```python
from build123d import *

# Parameters (mm, degrees)
F1_DEPTH      = 6.35
F2_R          = 2.54
F3_DEPTH      = 25.4
F3_DEPTH_BACK = 25.4


with BuildPart() as f1:
    # F0 (on Top) → F1 (new body)
    with BuildSketch(Plane.XY):
        with BuildLine():
            Line((-8.89, -12.7), (8.89, -12.7))
            ThreePointArc((8.89, -12.7), (11.584077, -11.584077), (12.7, -8.89))
            Line((12.7, -8.89), (12.7, 8.89))
            ThreePointArc((12.7, 8.89), (11.584077, 11.584077), (8.89, 12.7))
            Line((8.89, 12.7), (-8.89, 12.7))
            ThreePointArc((-8.89, 12.7), (-11.584077, 11.584077), (-12.7, 8.89))
            Line((-12.7, 8.89), (-12.7, -8.89))
            ThreePointArc((-12.7, -8.89), (-11.584077, -11.584077), (-8.89, -12.7))
        make_face()
    extrude(amount=F1_DEPTH)

    # F2 (on Top) → F3 (cut, two sides)
    with BuildSketch(Plane.XY) as f3_sk:
        with Locations((-6.336518, -6.325952)):
            Circle(F2_R)
        with Locations((6.331818, -6.326862)):
            Circle(F2_R)
        with Locations((6.324662, 6.333847)):
            Circle(F2_R)
        with Locations((-6.33241, 6.329887)):
            Circle(F2_R)
    extrude(amount=F3_DEPTH, mode=Mode.SUBTRACT)
    extrude(f3_sk.sketch, amount=-F3_DEPTH_BACK, mode=Mode.SUBTRACT)


solid = f1.part
```
Here's how the part is built. I have some questions about the finished solid (model axes, mm). Give positions to 0.01 mm unless a question says otherwise; leave off trailing zeros. Write each loop counter-clockwise with the first axis right and the second up, starting at its lowest first coordinate (ties: lowest second). Pieces come first, ordered by that corner, then holes.
(1) Imagine slicing it at B-B, the plane y = 8.5. Write out the boundary of the cut face in (x, z).
Output values:
outline: (-12.7, 0) - (-7.65, 0) - (-7.65, 6.35) - (-12.7, 6.35) - close; (-5.01, 0) - (5, 0) - (5, 6.35) - (-5.01, 6.35) - close; (7.65, 0) - (12.7, 0) - (12.7, 6.35) - (7.65, 6.35) - close
(2) Imagine slicing it at C-C, the plane z = 2.5. Write out the boundary of the cut face in (x, y).
Output values:
outline: (-12.7, -8.89) arc R3.81 ccw to (-8.89, -12.7) - (8.89, -12.7) arc R3.81 ccw to (12.7, -8.89) - (12.7, 8.89) arc R3.81 ccw to (8.89, 12.7) - (-8.89, 12.7) arc R3.81 ccw to (-12.7, 8.89) - close; hole circle Ø5.08 at (-6.34, -6.33); hole circle Ø5.08 at (-6.33, 6.33); hole circle Ø5.08 at (6.32, 6.33); hole circle Ø5.08 at (6.33, -6.33)
(3) If I drill on L1, parallel to Y at x = -5, z = 0.75; L2, parallel to X at y = -4, z = 3; L3, parallel to Y at x = 5.25, z = 3.75, over which ranges is the centre line in solid material (lowest first)?
Output values:
L1: y = -12.7 to -8.49, -4.17 to 4.17, 8.49 to 12.7
L2: x = -12.7 to -7.36, -5.32 to 5.31, 7.35 to 12.7
L3: y = -12.7 to -8.62, -4.03 to 4.03, 8.64 to 12.7
(4) Thinking about a two-plate mould opening in Y: for faces 1 (the face through (11.614, 11.554, 3.131)), 2 (the face through (4.3, 4.8, 3.1)), 3 (the face through (0, 0, 6.35)), which applies, pulls with the +Y half, pulls with the -Y half, needs draft (parallel to the pull), parting line crosses it, or undercut?
Output values:
face 1: pulls with the +Y half
face 2: undercut
face 3: needs draft
(5) Imagine slicing it at A-A, the plane x = 4.25. Write out the boundary of the cut face in (y, z).
Output values:
outline: (-12.7, 0) - (-7.78, 0) - (-7.78, 6.35) - (-12.7, 6.35) - close; (-4.87, 0) - (4.87, 0) - (4.87, 6.35) - (-4.87, 6.35) - close; (7.8, 0) - (12.7, 0) - (12.7, 6.35) - (7.8, 6.35) - close
